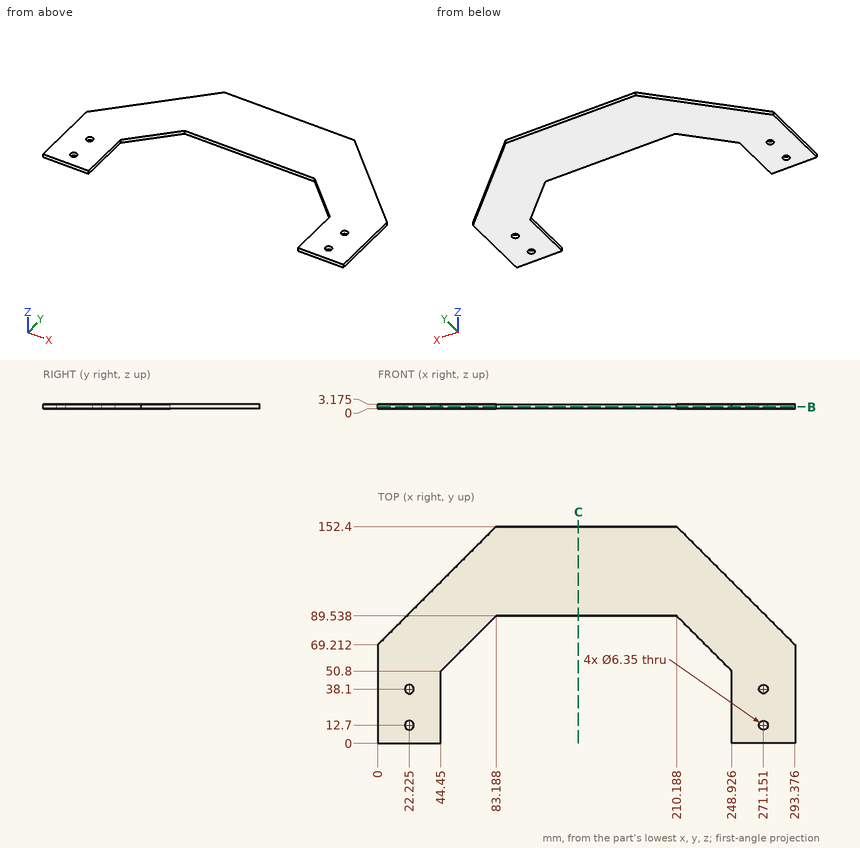
Could you check a few things on this drawing? It's one solid part, dimensions in mm from its lowest x, y, z. Round coordinates to 2 decimals unless told otherwise and drop trailing zeros. Order: outer loops, then holes, each group sorted by start corner. A loop starts at its lowest first (then second) coordinate and runs counter-clockwise, first axis right, second up. Notation, with made-up numbers: M -38,-37 L 0,-37 A29 cw 0,-11 Z; hole C 26.5,81.5 d11. An arc over 180 degrees is marked long. One line per item, written item: value.
(1) Imagine slicing it at C-C (x = 141). Write out the boundary of the cut face in (y, z) (1 decimal).
Ans:
outline: M 89.5,0 L 152.4,0 L 152.4,3.2 L 89.5,3.2 Z
(2) Imagine slicing it at B-B (z = 1.2). Count the separate pieces of the cut face and the enclosed holes in it, and give its area (3 significant figures).
Ans:
separate pieces: 1
enclosed holes: 4
area: 20,900 mm^2
(3) I need wall thicknesses on line 1 along X through (y, z) = (19.5, 0.7); line 2 along Y through (x, z) = (114, 0.8); line 3 along Y through (x, z) = (281.5, 3.05). Which ranges of each line are inside material? Lowest first, please. Write a range as from..to.
Ans:
line 1: x = 0..44.45, 248.93..293.38
line 2: y = 89.54..152.4
line 3: y = 0..81.09
